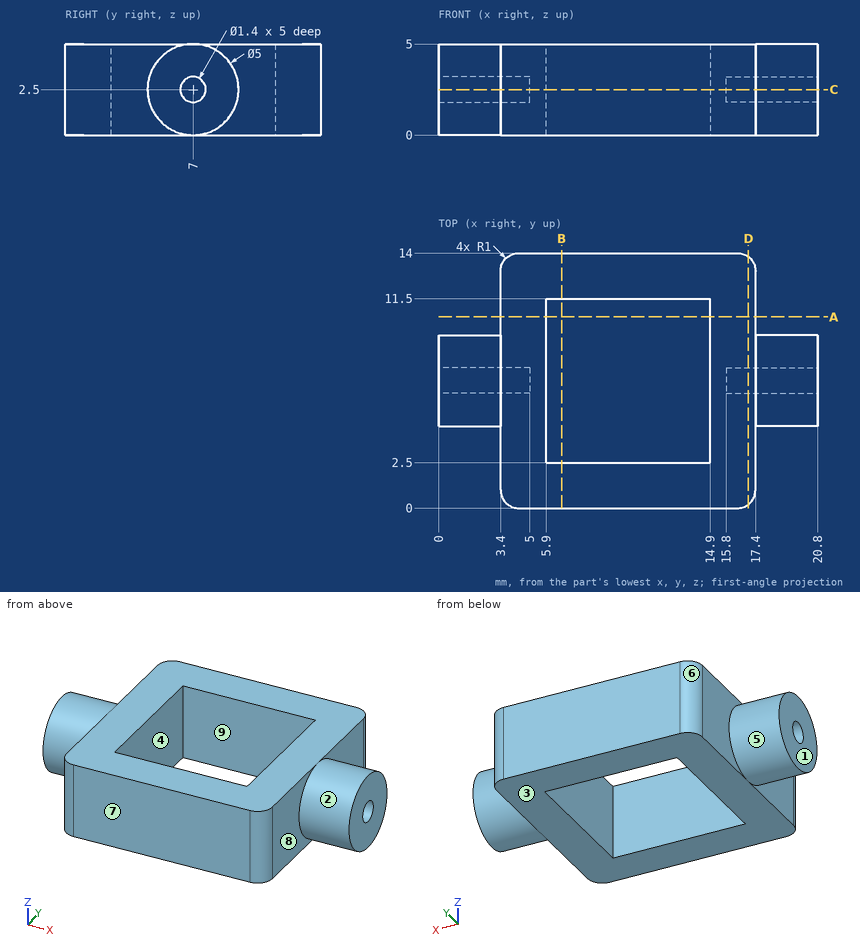
Answer from the drawing. Dimensions are ordinates in mm from the lowest x, y and z of the part. A direction names the side the tool comes from. Round coordinates to 2 decimals unless told otherwise and drop trailing zeros. Write each loop counter-clockwise with the first axis right and the second up, starting at its lowest first coordinate (ties: lowest second). Pieces come first, ordered by that corner, then holes. Notation, with made-up numbers: M 13,-31.5 L 33,-31.5 A22 ccw 33,-8.5 Z; hole C 13,73.5 d2. An arc over 180 degrees is marked long. Write each question's results on one line, items separated by ' | '. Start each with the question number.
Item 1: Given pin 1 Ø1.5 at (x, y) = (10.5, 10) entering from -Z; pin 2 Ø0.7 at (y, z) = (7, 2.5) entering from +X; pin 3 Ø1.1 at (y, z) = (7, 2.5) entering from -X; pin 4 Ø3 at (y, z) = (10.5, 0.5) entering from +X, each flat-ended and moving along its own axis, determine where each tip first touches the part or whether it passes through.
Item 2: Find section A-A on y = 10.5. Write down the section's boundary in (x, z).
Item 3: Find section C-C on z = 2.5. Write down the section's boundary in (x, y).
Item 4: The mould has two halves that part along Y. Classify the marked faces 6, 7, 8 and 9: +Y half, -Y half, draft (parallel to the pull), parting line (faces both ways), or undercut.
Item 5: Straight lines are drawn through the part: probe 1 along X at (y, z) = (4.5, 4.7); probe 2 along X at (y, z) = (5.5, 2); probe 3 along Y at (x, z) = (12.5, 4.75). For each, find the intervals that lie inside material, in ascending order.
Item 6: Which of the six approach directions +Z, -Z, +X, -X, +Y, -Y give full straight-line access (tool end or side, diameter ignored) to the marked faces 1, 2, 3, 4 and 5?
Item 7: Find section B-B on x = 6.75. Write down the section's boundary in (y, z).
Item 8: Find section D-D on x = 17. Write down the section's boundary in (y, z).
Answer block:
1) pin 1: passes through | pin 2: stops at x = 15.8 | pin 3: stops at x = 5 | pin 4: stops at x = 17.4
2) outline: M 3.4,0 L 5.9,0 L 5.9,5 L 3.4,5 Z; M 14.9,0 L 17.4,0 L 17.4,5 L 14.9,5 Z
3) outline: M 0,4.5 L 3.4,4.5 L 3.4,1 A1 ccw 4.4,0 L 16.4,0 A1 ccw 17.4,1 L 17.4,4.5 L 20.8,4.5 L 20.8,6.3 L 15.8,6.3 L 15.8,7.7 L 20.8,7.7 L 20.8,9.5 L 17.4,9.5 L 17.4,13 A1 ccw 16.4,14 L 4.4,14 A1 ccw 3.4,13 L 3.4,9.5 L 0,9.5 L 0,7.7 L 5,7.7 L 5,6.3 L 0,6.3 Z; hole M 5.9,2.5 L 14.9,2.5 L 14.9,11.5 L 5.9,11.5 Z
4) face 6: +Y half | face 7: -Y half | face 8: draft | face 9: undercut
5) probe 1: x = 3.4 to 5.9, 14.9 to 17.4 | probe 2: x = 0 to 5.9, 14.9 to 20.8 | probe 3: y = 0 to 2.5, 11.5 to 14
6) face 1: +Z, -Z, -X, +Y, -Y | face 2: +X | face 3: -Z, +X, -X, +Y, -Y | face 4: +Z, -Z | face 5: -X
7) outline: M 0,0 L 2.5,0 L 2.5,5 L 0,5 Z; M 11.5,0 L 14,0 L 14,5 L 11.5,5 Z
8) outline: M 0.2,0 L 13.8,0 L 13.8,5 L 0.2,5 Z; hole C 7,2.5 d1.4
